Design review of the part built by this model. Coordinates are the model's own, in mm. A direction names the side the tool comes from. Give positions to 0.01 mm unless a question says otherwise; leave off trailing zeros. Loops run counter-clockwise (first coordinate to the right, second up) from the corner with the lowest first, then second, coordinate; pieces in that order, holes last. Notation, with made-up numbers: (85.25, 83) -> (122.25, 83) arc R26 cw to (122.25, 104) -> close; hole circle Ø7 at (41, 59.5). An arc over 180 degrees is marked (long way). Answer in a Markdown table with one row per item. Add a question column.
(1) Consider section C-C on y = 3.15. Count the separate pieces of the cut face and the enclosed holes in it, then the cut area to 3 significant figures.
(2) For pin 1 (8 mm diameter, centred on x = -32, z = -33, fed in from +Y); pin 2 (1 mm diameter, centred on y = 1, z = -40, fed in from +X); pin 3 (1.5 mm diameter, centred on x = -53, y = 3.5, fed in from -Z), all flat-tipped, find the tip position at first contact; note any pin that passes through.
(3) Consider section B-B on z = -6.5. Write out the cut boundary in (x, y), then the cut area to 3 significant figures.
(4) For faces 3 (the flat face through (0.321, 2.465, -14.607)), 4 (the flat face through (-34, 0, -4)), list the 3-axis set-ups (+Z, -Z, +X, -X, +Y, -Y) from which the entire face can be reached by the end or side of a thin tool; tool diameter is ignored.
(5) Draft analysis for pull direction Z (two halves, no side actions). For faces 1 (the flat face through (-21.528, 2.465, 11.529)), 2 (the flat face through (-56, 5.199, -36)), state which applies: +Z half, -Z half, draft (parallel to the pull), parting line (faces both ways), or undercut.
(6) Consider section A-A on x = -47. Write out the cut boundary in (y, z).
(7) For line 1 (Z direction, x = -32.5, y = 0.8); line 2 (Z direction, x = 4, y = 3.2); line 3 (Z direction, x = -3.5, y = 3.4), list the stretches that pass through material, from the lowest coordinate up.
Autodesk Fusion 360 part; units mm, degrees
sketch "草图1" plane through (0, 0, 0) normal (0, 1, 0) x (1, 0, 0)
  point P0 (-25, 10)
sketch "草图2" plane through (0, 0, 0) normal (0, 1, 0) x (1, 0, 0)
  circle A0 centre (-25, 10) radius 40.6099
  line L0 (-13.7666, 45.8931) -> (-29.5688, 24.8235)
  line L1 (-15.0058, 39.2409) -> (-26.584, 23.8033)
  line L2 (-29.5688, 24.8235) -> (-54.4904, 33.3414)
  line L3 (-31.4615, 22.3) -> (-49.7214, 28.541)
  line L4 (-49.7214, 28.541) -> (-38.6172, 12.759)
  line L5 (-31.4615, 22.3) -> (-38.6172, 12.759)
  line L6 (-40.5098, 10.2355) -> (-56.312, -10.8341)
  line L7 (-55.6651, 31.7752) -> (-40.5098, 10.2355)
  line L8 (-28.4766, 21.2798) -> (-36.802, 10.1792)
  line L9 (-38.6947, 7.6557) -> (-50.2729, -7.7819)
  line L10 (-50.2729, -7.7819) -> (-31.8319, -2.0981)
  line L11 (-38.6947, 7.6557) -> (-31.8319, -2.0981)
  line L12 (-30.0168, -4.6779) -> (-14.8615, -26.2176)
  line L13 (-55.1855, -12.4353) -> (-30.0168, -4.6779)
  line L14 (-36.802, 10.1792) -> (-28.8175, -1.169)
  line L15 (-27.0023, -3.7488) -> (-15.8981, -19.5309)
  line L16 (-15.8981, -19.5309) -> (-15.6052, -0.2361)
  line L17 (-28.8175, -1.169) -> (-15.5573, 2.918)
  line L18 (-12.5428, 3.8471) -> (5.8981, 9.5309)
  line L19 (-12.9906, -25.641) -> (-12.5907, 0.693)
  line L20 (-27.0023, -3.7488) -> (-15.6052, -0.2361)
  line L21 (-12.5907, 0.693) -> (12.578, 8.4504)
  line L22 (5.8981, 9.5309) -> (-12.3618, 15.7719)
  line L23 (-15.3466, 16.7921) -> (-28.4766, 21.2798)
  line L24 (12.6077, 10.408) -> (-12.3139, 18.9259)
  line L25 (-15.2987, 19.9461) -> (-26.584, 23.8033)
  line L26 (-15.5573, 2.918) -> (-15.3466, 16.7921)
  line L27 (-15.2987, 19.9461) -> (-15.0058, 39.2409)
  line L28 (-12.5428, 3.8471) -> (-12.3618, 15.7719)
  line L29 (-12.3139, 18.9259) -> (-11.914, 45.2599)
  arc A1 (-13.7666, 45.8931) -> (-54.4904, 33.3414) centre (-25, 10) ccw
  arc A2 (-55.6651, 31.7752) -> (-56.312, -10.8341) centre (-25, 10) ccw
  arc A3 (-55.1855, -12.4353) -> (-14.8615, -26.2176) centre (-25, 10) ccw
  arc A4 (-12.9906, -25.641) -> (12.578, 8.4504) centre (-25, 10) ccw
  arc A5 (12.6077, 10.408) -> (-11.914, 45.2599) centre (-25, 10) ccw
  point P0 (-15.0058, 39.2409)
  point P1 (-50.2729, -7.7819)
  point P2 (5.8981, 9.5309)
  point P3 (-49.7214, 28.541)
  point P4 (-25, 10)
extrude "拉伸1" add sketch "草图2" along normal blind 5 makes body 1
sketch "草图3" plane through (0, 0, 0) normal (0, 1, 0) x (1, 0, 0)
sketch "草图4" plane through (0, 0, 0) normal (0, 1, 0) x (1, 0, 0)
sketch "草图5" plane through (0, 0, 0) normal (0, 1, 0) x (1, 0, 0)
sketch "草图6" plane through (0, 0, 0) normal (0, 1, 0) x (1, 0, 0)
  circle A0 centre (40, -20) radius 2.5
  circle A1 centre (40, -20) radius 4
  dimension "d5" = 5
  dimension "d6" = 8
extrude "拉伸2" add sketch "草图6" along normal blind 5 separate body makes body 2
move_body "移动1" bodies 2 to x (1, 0, 0) y (0, 1, 0) z (0, 0, 1) at (-108.6235, 0.1986, -28.1984)
move_body "移动2" bodies 2 to x (1, 0, 0) y (0, 1, 0) z (0, 0, 1) at (9.1347, 0, -27.4041)
move_body "移动3" bodies 2 to x (1, 0, 0) y (0, 1, 0) z (0, 0, 1) at (-0.1986, 0, -0.9929)
move_body "移动4" bodies 2 to x (1, 0, 0) y (0, 1, 0) z (0, 0, 1) at (0.3972, 0, 0.7943)
move_body "移动5" bodies 2 to x (1, 0, 0) y (0, 1, 0) z (0, 0, 1) at (0.3972, 0, 0)
move_body "移动6" bodies 2 to x (1, 0, 0) y (0, 1, 0) z (0, 0, 1) at (-0.7943, 0, 0)
move_body "移动7" bodies 2 to x (1, 0, 0) y (0, 1, 0) z (0, 0, 1) at (0.7943, 0, -0.5957)
combine "合并1" operation add target body 1 tool bodies 2
Values follow:
| question | item | result |
|---|---|---|
| 1 | separate pieces | 1 |
| 1 | enclosed holes | 12 |
| 1 | area | 1,720 mm2 |
| 2 | pin 1 | through |
| 2 | pin 2 | x = 2.91 |
| 2 | pin 3 | z = -40.11 |
| 3 | outline | (-65.46, 0) -> (-62.45, 0) -> (-62.45, 5) -> (-65.46, 5) -> close; (-43.31, 0) -> (-39.56, 0) -> (-39.56, 5) -> (-43.31, 5) -> close; (-37.88, 0) -> (-34.21, 0) -> (-34.21, 5) -> (-37.88, 5) -> close; (-15.5, 0) -> (-12.5, 0) -> (-12.5, 5) -> (-15.5, 5) -> close; (-3.94, 0) -> (6.25, 0) -> (6.25, 5) -> (-3.94, 5) -> close; (12.45, 0) -> (15.46, 0) -> (15.46, 5) -> (12.45, 5) -> close |
| 3 | area | 133 mm2 |
| 4 | face 3 | +Y, -Y |
| 4 | face 4 | +Z, -Z, +X, -X, -Y |
| 5 | face 1 | undercut |
| 5 | face 2 | draft |
| 6 | outline | (0, -44.13) -> (5, -44.13) -> (5, -40.5) -> (0, -40.5) -> close; (0, -30.78) -> (5, -30.78) -> (5, -27.61) -> (0, -27.61) -> close; (0, -24.67) -> (5, -24.67) -> (5, -19.46) -> (0, -19.46) -> close; (0, -1.58) -> (5, -1.58) -> (5, 3.42) -> (0, 3.42) -> close; (0, 6.77) -> (5, 6.77) -> (5, 9.91) -> (0, 9.91) -> close; (0, 20.5) -> (5, 20.5) -> (5, 24.13) -> (0, 24.13) -> close |
| 7 | line 1 | -49.91 to -46.85, -25.83 to -22.65, -20.92 to -15.92, -4.06 to 1.15, 2.3 to 5.44, 26.85 to 29.91 |
| 7 | line 2 | -38.43 to -33.95, -13.35 to -10.18, -8.95 to -5.81, 13.95 to 18.43 |
| 7 | line 3 | -44.45 to -40.86, -15.91 to -12.74, -6.63 to -3.49, 20.86 to 24.45 |
